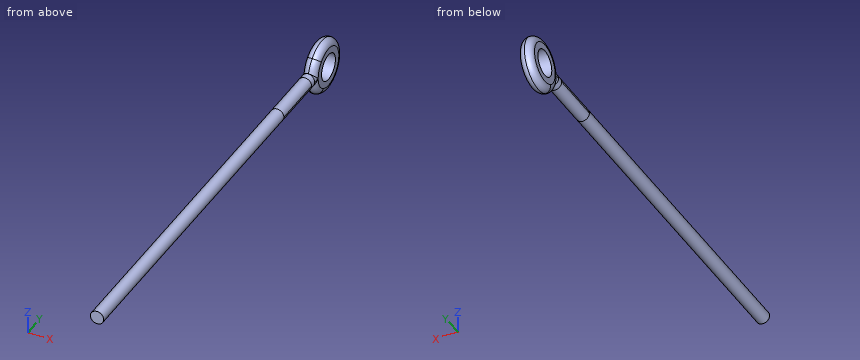
```python
from build123d import *

# Parameters (mm, degrees)
SKETCH1_R                = 12.626048476
SKETCH1_R_2              = 6.35
BOSS_EXTRUDE1_DEPTH      = 6.35
BOSS_EXTRUDE2_DEPTH      = 6.35
SKETCH4_R                = 3.175
BOSS_EXTRUDE3_DEPTH      = 50.8
CUT_EXTRUDE1_START       = -6.35
CUT_EXTRUDE1_DEPTH       = 6.35
SKETCH7_R                = 3.175
BOSS_EXTRUDE4_DEPTH      = 57.15
SKETCH7_2_R              = 3.175
CUT_EXTRUDE2_DEPTH       = 25.4
FILLET1_R                = 3.175
BOSS_EXTRUDE5_DEPTH      = 139.7
BOSS_EXTRUDE5_DEPTH_BACK = 25.4
SKETCH7_3_R              = 3.175


with BuildPart() as part:
    # Sketch1 → Boss-Extrude1 (new body)
    with BuildSketch(Plane(origin=(0, 0, 0), x_dir=(0, 0, -1), z_dir=(1, 0, 0))):
        Circle(SKETCH1_R)
        Circle(SKETCH1_R_2, mode=Mode.SUBTRACT)
    extrude(amount=BOSS_EXTRUDE1_DEPTH)

    # Sketch3 → Boss-Extrude2 (add)
    with BuildSketch(Plane(origin=(6.35, 0, 0), x_dir=(0, 0, -1), z_dir=(1, 0, 0))):
        Polygon((-8.994798287, -8.860626609), (-8.994798287, -15.452306957), (10.798615768, -15.452306957), (10.798615768, -6.542705681), (-8.994798287, -6.542705681), align=None)
    extrude(amount=-BOSS_EXTRUDE2_DEPTH)

    # Sketch4 → Boss-Extrude3 (add)
    with BuildSketch(Plane.XZ.offset(15.452306957)):
        with Locations(Location((3.175, 0, 0), (0, 0, 180))):
            Circle(SKETCH4_R)
    extrude(amount=BOSS_EXTRUDE3_DEPTH)

    # Sketch5 → Cut-Extrude1 (cut)
    with BuildSketch(Plane(origin=(6.35, 0, 0), x_dir=(0, 0, -1), z_dir=(1, 0, 0)).offset(CUT_EXTRUDE1_START)):
        with BuildLine():
            Line((-8.994798287, -8.860626609), (-8.994798287, -15.452306957))
            Line((-8.994798287, -15.452306957), (10.798615768, -15.452306957))
            Line((10.798615768, -15.452306957), (10.798615768, -6.542705681))
            ThreePointArc((10.798615768, -6.542705681), (1.46854647, -12.540353719), (-8.994798287, -8.860626609))
        make_face()
    extrude(amount=CUT_EXTRUDE1_DEPTH, mode=Mode.SUBTRACT)


with BuildPart() as cut_extrude1_piece_1:
    # of the separate pieces the step leaves, piece 1, a body of its own (cut_extrude1_pieces)
    add(part.part.solids().sort_by_distance((0, -6.542705681, -10.798615768))[0])



with BuildPart() as cut_extrude1_piece_2:
    # of the separate pieces the step leaves, piece 2, a body of its own (cut_extrude1_pieces)
    add(part.part.solids().sort_by_distance((0, -15.452306957, 0))[0])


with BuildPart() as cut_extrude1_piece_1_1:
    add(cut_extrude1_piece_1.part)

    add(cut_extrude1_piece_2.part)  # Boss-Extrude4 merges Cut-Extrude1 piece 2
    # Sketch7 → Boss-Extrude4 (add)
    with BuildSketch(Plane.XZ.offset(66.252306957)):
        with Locations((3.175, 0)):
            Circle(SKETCH7_R)
    extrude(amount=-BOSS_EXTRUDE4_DEPTH)

    # Sketch7<2> → Cut-Extrude2 (cut)
    with BuildSketch(Plane.XZ.offset(66.252306957)):
        with Locations((3.175, 0)):
            Circle(SKETCH7_2_R)
    extrude(amount=-CUT_EXTRUDE2_DEPTH, mode=Mode.SUBTRACT)

    # Fillet1
    # the kernel refuses this fillet: 3.175 mm, written as the material it takes off along each edge
    with BuildSketch(Plane(origin=(6.35, 0, 0), x_dir=(0, -0.7017735299957855, 0.7124001071008161), z_dir=(0, -0.7124001071008161, -0.7017735299957855))) as fillet1_piece_1:
        with BuildLine():
            CenterArc((12.626048476 - FILLET1_R, FILLET1_R), FILLET1_R, 270, 90)
            Line((12.626048476 - FILLET1_R, 0), (12.626048476, 0))
            Line((12.626048476, 0), (12.626048476, FILLET1_R))
        make_face()
    revolve(axis=Axis((6.35, 0, 0), (-1, 0, 0)), revolution_arc=255.78045899, mode=Mode.SUBTRACT)
    with BuildSketch(Plane(origin=(0, 0, 0), x_dir=(0, -0.5181910787843432, -0.855264874684047), z_dir=(0, -0.855264874684047, 0.5181910787843432))) as fillet1_piece_2:
        with BuildLine():
            CenterArc((12.626048476 - FILLET1_R, FILLET1_R), FILLET1_R, 270, 90)
            Line((12.626048476 - FILLET1_R, 0), (12.626048476, 0))
            Line((12.626048476, 0), (12.626048476, FILLET1_R))
        make_face()
    revolve(axis=Axis((0, 0, 0), (1, 0, 0)), revolution_arc=255.78045899, mode=Mode.SUBTRACT)
    with BuildSketch(Plane(origin=(0, 0, 0), x_dir=(0, -0.5181910787843435, -0.8552648746840469), z_dir=(0, 0.8552648746840469, -0.5181910787843435))) as fillet1_piece_3_section:
        with BuildLine():
            CenterArc((12.626048476 - FILLET1_R, -FILLET1_R), FILLET1_R, 0, 90)
            Line((12.626048476 - FILLET1_R, 0), (12.626048476, 0))
            Line((12.626048476, 0), (12.626048476, -FILLET1_R))
        make_face()
    fillet1_piece_3 = revolve(axis=Axis((0, 0, 0), (-1, 0, 0)), revolution_arc=58.789009325, mode=Mode.PRIVATE)
    fillet1_piece_3 = fillet1_piece_3 - Plane(origin=(3.175, -9.611252213, 0), x_dir=(1, 0, 0), z_dir=(0, -1, 0)) * Cylinder(3.175, 51, mode=Mode.PRIVATE)
    add(fillet1_piece_3, mode=Mode.SUBTRACT)
    with BuildSketch(Plane(origin=(0, 0, 0), x_dir=(0, -1, 0), z_dir=(0, 0, -1))) as fillet1_piece_4_section:
        with BuildLine():
            CenterArc((12.626048476 - FILLET1_R, -FILLET1_R), FILLET1_R, 0, 90)
            Line((12.626048476 - FILLET1_R, 0), (12.626048476, 0))
            Line((12.626048476, 0), (12.626048476, -FILLET1_R))
        make_face()
    fillet1_piece_4 = revolve(axis=Axis((0, 0, 0), (-1, 0, 0)), revolution_arc=45.430531685, mode=Mode.PRIVATE)
    fillet1_piece_4 = fillet1_piece_4 - Plane(origin=(3.175, -10.439695548, 0), x_dir=(1, 0, 0), z_dir=(0, -1, 0)) * Cylinder(3.175, 51, mode=Mode.PRIVATE)
    add(fillet1_piece_4, mode=Mode.SUBTRACT)
    with BuildSketch(Plane(origin=(6.35, 0, 0), x_dir=(0, -1, 0), z_dir=(0, 0, -1))) as fillet1_piece_5_section:
        with BuildLine():
            CenterArc((12.626048476 - FILLET1_R, FILLET1_R), FILLET1_R, 270, 90)
            Line((12.626048476 - FILLET1_R, 0), (12.626048476, 0))
            Line((12.626048476, 0), (12.626048476, FILLET1_R))
        make_face()
    fillet1_piece_5 = revolve(axis=Axis((6.35, 0, 0), (-1, 0, 0)), revolution_arc=45.430531685, mode=Mode.PRIVATE)
    fillet1_piece_5 = fillet1_piece_5 - Plane(origin=(3.175, -10.439696502, 0), x_dir=(1, 0, 0), z_dir=(0, -1, 0)) * Cylinder(3.175, 51, mode=Mode.PRIVATE)
    add(fillet1_piece_5, mode=Mode.SUBTRACT)
    with BuildSketch(Plane(origin=(6.35, 0, 0), x_dir=(0, -0.5181910787843435, -0.8552648746840469), z_dir=(0, 0.8552648746840469, -0.5181910787843435))) as fillet1_piece_6_section:
        with BuildLine():
            CenterArc((12.626048476 - FILLET1_R, FILLET1_R), FILLET1_R, 270, 90)
            Line((12.626048476 - FILLET1_R, 0), (12.626048476, 0))
            Line((12.626048476, 0), (12.626048476, FILLET1_R))
        make_face()
    fillet1_piece_6 = revolve(axis=Axis((6.35, 0, 0), (-1, 0, 0)), revolution_arc=58.789009325, mode=Mode.PRIVATE)
    fillet1_piece_6 = fillet1_piece_6 - Plane(origin=(3.175, -9.611252422, 0), x_dir=(1, 0, 0), z_dir=(0, -1, 0)) * Cylinder(3.175, 51, mode=Mode.PRIVATE)
    add(fillet1_piece_6, mode=Mode.SUBTRACT)

    # Sketch7<3> → Boss-Extrude5 (add, two sides: drawn at the far end of the back side and taken through both)
    with BuildSketch(Plane.XZ.offset(66.252306957).offset(-BOSS_EXTRUDE5_DEPTH_BACK)):
        with Locations(Location((3.175, 0, 0), (0, 0, 270))):
            Circle(SKETCH7_3_R)
    extrude(amount=BOSS_EXTRUDE5_DEPTH + BOSS_EXTRUDE5_DEPTH_BACK)


solid = cut_extrude1_piece_1_1.part
```
Can you work these out from the model? Positions are in its coordinate system, mm. Coordinates: 2 decimals unless noted, no trailing zeros. Loops run counter-clockwise (first coordinate to the right, second up) from the corner with the lowest first, then second, coordinate; pieces in that order, holes last. Notation, with made-up numbers: (17, -22) -> (21, -22) arc R24 ccw to (21, 11) -> close; hole circle Ø5 at (-1.75, 62.5). An arc over 180 degrees is marked (long way). Put each result on its own line as item: value. Start each with the question number.
Q1. I want a section at A-A (y = 0). Write out the boundary of the cut face in (x, z) (3 decimals).
Q2. I want a section at B-B (x = 1.75). Write out the boundary of the cut face in (y, z).
Q3. If I drill on line 1 (Y direction, x = 3.25, z = 0); line 2 (Y direction, x = 2.25, z = 5.75); line 3 (X direction, y = -135.5, z = -0.25), over which ranges is the centre line in solid material (lowest first)? Write a range as [from, to].
Q4. I'm going to push flat-ended pins straight in: P1, Ø1, axis at x = 5.5, y = -133, coming from the -Z side; P2, Ø1.5, axis at x = 2.5, z = 7.5, coming from the -Y side. Where does each tip first touch, or does it pass through?
Q5. I want a section at C-C (y = -182). Write out the boundary of the cut face in (x, z) (3 decimals).
Taken from the geometry:
1. outline: (0, -9.451) arc R3.175 ccw to (6.35, -9.451) -> (6.35, -6.35) -> (0, -6.35) -> close; (0, 6.35) -> (6.35, 6.35) -> (6.35, 9.451) arc R3.175 ccw to (0, 9.451) -> close
2. outline: (-205.95, -2.84) -> (-11.96, -2.84) arc R12.29 ccw (long way) to (-11.96, 2.84) -> (-205.95, 2.84) -> close; hole circle Ø12.7 at (0, 0)
3. line 1: y = [-205.95, -6.35], [6.35, 12.63]
3. line 2: y = [-11.09, -2.69], [2.69, 11.09]
3. line 3: x = [0.01, 6.34]
4. P1: stops at z = -2.6
4. P2: stops at y = -10.61
5. outline: circle Ø6.35 at (3.175, 0)
